Source: three-view drawing plus pictorial views. Frame: mm from the lowest corner of the part. Give positions to 0.01 mm unless a question says otherwise; leave off trailing zeros. Order: outer loops, then holes, each group sorted by start corner. A loop starts at its lowest first (then second) coordinate and runs counter-clockwise, first axis right, second up.
1) Section C-C, the plane z = 13. Return loops of the section in (x, y), plus the area to 3 significant figures.
2) First-contact query: P1, Ø3.5, axis at x = 2, z = 13, coming from the -Y side. Flat tip, straight axial feed; report the tip coordinate or a pass-through.
3) Section A-A, the plane x = 2. Return loops of the section in (y, z).
4) Material intervals for line 1 (Z direction, x = 2, y = 3); line 2 (Z direction, x = 1, y = 6.5); line 3 (X direction, y = 7.5, z = 13), sorted ascending.
5) Section B-B, the plane y = 6.5. Return loops of the section in (x, z), plus the area to 3 significant figures.
6) Draft query along Z for the marked faces 1, 2, 3 and 4. Return one class per face: released by +Z, released by -Z, zero draft, split by the parting line, or undercut.
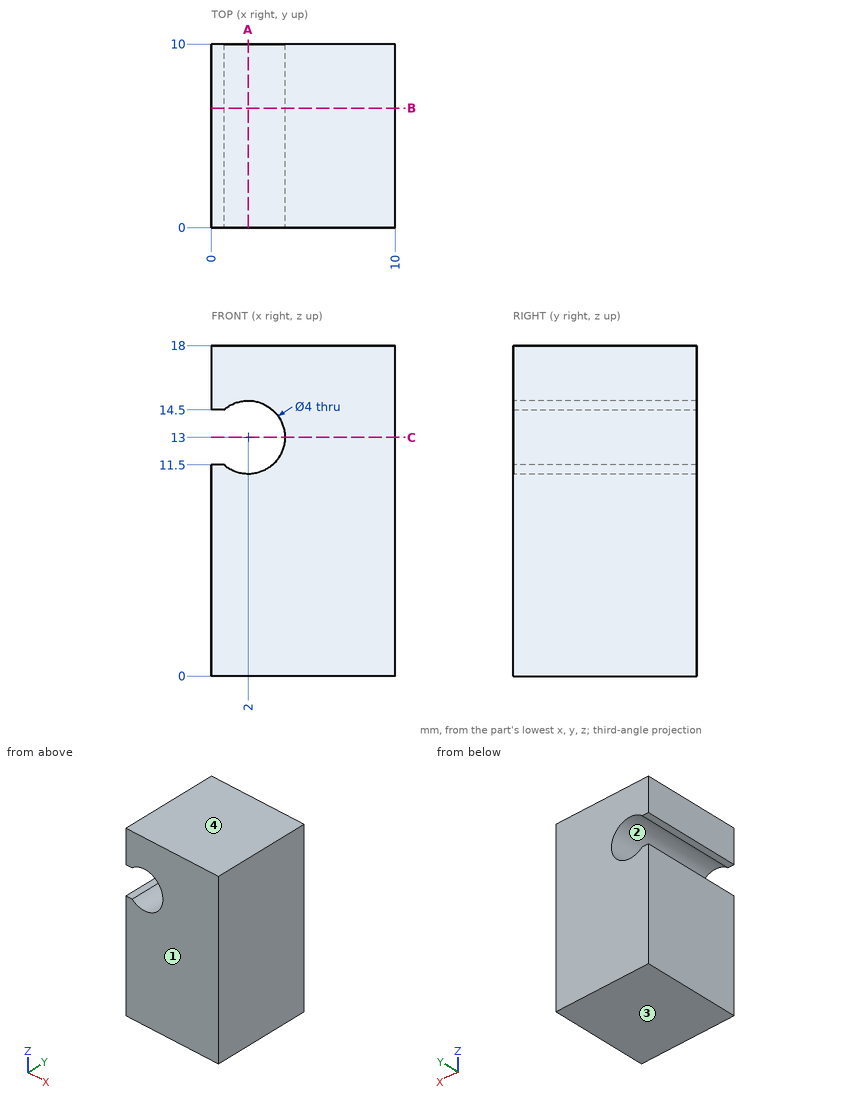
From the geometry:
1. outline: (4, 0) - (10, 0) - (10, 10) - (4, 10) - close
1. area: 60.0 mm2
2. P1: passes through
3. outline: (0, 0) - (10, 0) - (10, 11) - (0, 11) - close; (0, 15) - (10, 15) - (10, 18) - (0, 18) - close
4. line 1: z = 0 to 11, 15 to 18
4. line 2: z = 0 to 11.27, 14.73 to 18
4. line 3: x = 4 to 10
5. outline: (0, 0) - (10, 0) - (10, 18) - (0, 18) - (0, 14.5) - (0.68, 14.5) arc R2 cw (long way) to (0.68, 11.5) - (0, 11.5) - close
5. area: 167 mm2
6. face 1: zero draft
6. face 2: undercut
6. face 3: released by -Z
6. face 4: released by +Z
